Geometry: final body of the model. Coordinates: model frame, mm. A direction names the side the tool comes from. Give positions to 0.01 mm unless a question says otherwise; leave off trailing zeros. Loops run counter-clockwise (first coordinate to the right, second up) from the corner with the lowest first, then second, coordinate; pieces in that order, holes last. Notation, with made-up numbers: M 85,-30 L 89,-30 A30 ccw 89,7 Z; hole C 13,20.5 d9. An arc over 180 degrees is marked long. Put each result on its own line as item: value.
```python
from build123d import *

# Parameters (mm, degrees)
F1_DEPTH    = 7.62
F2_T1_DEPTH = 80.1722009782
F3_R        = 2.54
F4_DEPTH    = 5.08


# Not quite as in the source:
# - a fillet or chamfer that OpenCascade refuses, or shapes differently, is made with other operations: its cross-section is extruded or revolved along the edge and cut away or added


with BuildPart() as f1:
    # F0 (on Front) → F1 (new body)
    with BuildSketch(Plane.XZ):
        Polygon((-48.8362722099, 5.4695218146), (-48.8362722099, -19.9304781854), (103.5160953464, -16.1204781854), (103.5160953464, 1.6595218146), align=None)
    extrude(amount=F1_DEPTH)

    # F2: fillet of radius 11.684 on 1 edges, made by hand

    # F2_s2 → F2_t1 (cut)
    with BuildSketch(Plane.XY.offset(-47.3165786745)):
        with BuildLine():
            ThreePointArc((-48.8362722099, 0), (-44.5538661868, -5.527653455), (-37.8818320142, -7.62))
            Line((-37.8818320142, -7.62), (-48.8362722099, -7.62))
            Line((-48.8362722099, -7.62), (-48.8362722099, 0))
        make_face()
    extrude(amount=F2_T1_DEPTH, mode=Mode.SUBTRACT)

    # F3 (on face) → F4 (cut)
    with BuildSketch(Plane(origin=(0, 0, 0), x_dir=(-1, 0, 0), z_dir=(0, 1, 0))):
        with Locations((40.8820770681, -7.3196464218)):
            Circle(F3_R)
    extrude(amount=-F4_DEPTH, mode=Mode.SUBTRACT)


solid = f1.part
```
Item 1: Pin query (flat end, axial travel): pin 1 Ø6 at (x, z) = (81.5, -10) entering from +Y; pin 2 Ø4.5 at (x, z) = (-40.88, -7.32) entering from -Y; pin 3 Ø1.5 at (x, y) = (17, -4) entering from +Z; pin 4 Ø4 at (x, y) = (34.5, -6.5) entering from +Z. Return the tip coordinate at first contact, or that it passes through.
Output values:
pin 1: y = 0
pin 2: y = -7.6
pin 3: z = 3.84
pin 4: z = 3.44
Item 2: Section B-B on z = -3. Output: boundary loops of the cut face in (x, y), then the cut area to 3 significant figures.
Output values:
outline: M -48.84,0 A11.68 ccw -37.88,-7.62 L 103.52,-7.62 L 103.52,0 Z
area: 1,140 mm²
Item 3: Mould query, pull axis Z, two halves, no side actions, for faces 1 (the flat face through (-41, -5.08, -7)), 2 (the flat face through (26, 0, -7)). Classes: pulls with the +Z half, pulls with the -Z half, needs draft (parallel to the pull), parting line crosses it, or undercut.
Output values:
face 1: undercut
face 2: needs draft
Item 4: Section C-C on x = 32. Output: boundary loops of the cut face in (y, z).
Output values:
outline: M -7.62,-17.91 L 0,-17.91 L 0,3.45 L -7.62,3.45 Z
Item 5: Set-up query: faces 3 (the cylindrical face through (-44.635, -5.471, -7.408)), 4 (the cylindrical face through (-43.305, -2.504, -6.557)). Return all of +Z, -Z, +X, -X, +Y, -Y with unobstructed straight access to the full face (end or side cutting, diameter ignored); none if empty.
Output values:
face 3: +Z, -Z, -X, -Y
face 4: +Y
Item 6: Section A-A on y = -3.25. Output: boundary loops of the cut face in (x, z), then the cut area to 3 significant figures.
Output values:
outline: M -46.99,-19.88 L 103.52,-16.12 L 103.52,1.66 L -46.99,5.42 Z; hole C -40.88,-7.32 d5.08
area: 3,220 mm²
Item 7: Line query: probe 1 along X at (y, z) = (-3.5, -8.75); probe 2 along Z at (x, y) = (50, -5.5); probe 3 along X at (y, z) = (-5, -1.75). Output: solid intervals per line, ascending. Write a range as [from, to].
Output values:
probe 1: [-46.79, -42.98], [-38.78, 103.52]
probe 2: [-17.46, 3]
probe 3: [-45.25, 103.52]
